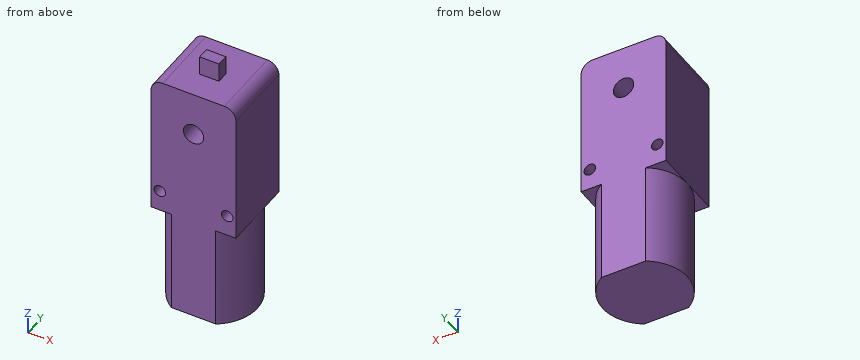
Autodesk Inventor part; units mm, degrees
ref_plane "YZ Plane" through (0, 0, 0) normal (1, 0, 0) x (0, 1, 0)
ref_plane "XZ Plane" through (0, 0, 0) normal (0, 1, 0) x (-1, 0, 0)
ref_plane "XY Plane" through (0, 0, 0) normal (0, 0, 1) x (1, 0, 0)
sketch "Sketch1" plane through (0, 0, 0) normal (0, 1, 0) x (-1, 0, 0)
  line L0 (0, 0) -> (-22, 0)
  line L1 (-22, 0) -> (-22, -37)
  line L2 (-22, -37) -> (0, -37)
  line L3 (0, -37) -> (0, 0)
  line L4 (-11, -37) -> (-11, 0) construction
  circle A0 centre (-11, -11.4) radius 2.65
  circle A1 centre (-19.75, -31.5) radius 1.5
  circle A2 centre (-2.25, -31.5) radius 1.5
  dimension "gearboxWidth" = 22
  dimension "gearboxLength" = 37
  dimension "shaftDiameter" = 5.3
  dimension "shaftCenterToBottom" = 11.4
  dimension "mountHolesDiameter" = 3
  dimension "mountHolesCenterToCenter" = 17.5
  dimension "mountHolesCenterToEdge" = 5.5
extrude "Extrusion1" add sketch "Sketch1" along normal blind 19
sketch "Sketch2" plane through (22, 0, -37) normal (0, 0, -1) x (-1, 0, 0)
  line L0 (0, 19) -> (22, 19)
  line L1 (11, 19) -> (11, 0) construction
  line L2 (0, 0) -> (22, 0)
  ellipse E0 centre (11, 9.5) end of major axis (22, 9.5) minor radius 11.1399 (16.7448, 0) -> (16.7448, 19) ccw
  ellipse E1 centre (11, 9.5) end of major axis (22, 9.5) minor radius 11.1399 (5.2552, 19) -> (5.2552, 0) ccw
  line L3 (5.2552, 19) -> (16.7448, 19)
  line L4 (5.2552, 0) -> (16.7448, 0)
extrude "Extrusion2" add sketch "Sketch2" along normal blind 27
fillet "Fillet1" radius 3 2 edges at (0, 9.5, 0) (22, 9.5, 0)
sketch "Sketch3" plane through (0, 0, 0) normal (0, 0, 1) x (1, 0, 0)
  line L0 (0, 0) -> (22, 0)
  line L1 (16.7448, 0) -> (5.2552, 0)
  line L2 (11, 0) -> (11, 18.9763) construction
  line L3 (8.5, 10) -> (8.5, 7)
  line L4 (8.5, 7) -> (13.5, 7)
  line L5 (13.5, 7) -> (13.5, 10)
  line L6 (13.5, 10) -> (8.5, 10)
  line L7 (8.5, 10) -> (13.5, 7) construction
  line L8 (8.5, 7) -> (13.5, 10) construction
  point P0 (11, 8.5)
  dimension "gearboxTabWidth" = 5
  dimension "gearboxTabHeight" = 3
  dimension "gearboxTabOffsetFromBottom" = 7
extrude "Extrusion3" add sketch "Sketch3" along normal blind 5
properties part number "Yellow_Motor"
Here's how the part is built. I have some questions about the finished solid (model axes, mm). Coordinates: 2 decimals unless noted, no trailing zeros. Order: outer loops, then holes, each group sorted by start corner. A loop starts at its lowest first (then second) coordinate and runs counter-clockwise, first axis right, second up. Notation, with made-up numbers: M 46.5,46.5 L 88.5,46.5 A29 cw 88.5,72.5 Z; hole C -20.75,30 d11. An arc over 180 degrees is marked long. Answer as a JSON object with one key per item and string values. Group by question number.
(1) Suppose I cut it at D-D, the plane x = 6. Please give me the cut outline in (y, z).
(2) For pin 1 (5 mm diameter, centred on x = 16, y = 12, fed in from +Z); pin 2 (2.5 mm diameter, centred on y = 8.5, z = 3, fed in from +X); pin 3 (2.5 mm diameter, centred on x = 2.25, z = -31.5, fed in from +Y); pin 4 (1.5 mm diameter, centred on y = 8.5, z = 2, fed in from -X), each with a flat end and sliding along its axis, tell me the tip position at first contact or that it passes through.
(3) Suppose I cut it at C-C, the plane y = 2.5. State how many separate pieces and enclosed holes the cut face has, then the cut area to 3 significant figures.
(4) Suppose I cut it at A-A, the plane z = -31.5. Please give me the cut outline in (x, y).
(5) Suppose I cut it at B-B, the plane x = 11. Please give me the cut outline in (y, z), then the cut area to 3 significant figures.
(6) I need wall thicknesses on probe 1 along X at (y, z) = (15.75, -11.5); probe 2 along Z at (x, y) = (11, 5.25); probe 3 along Z at (x, y) = (11, 7.25). Which ranges of each line are inside material? Lowest first, please.
Values found:
{
 "1": {"outline": "M 0,-64 L 19,-64 L 19,0 L 0,0 Z"},
 "2": {"pin 1": "stops at z = 0", "pin 2": "stops at x = 13.5", "pin 3": "passes through", "pin 4": "stops at x = 8.5"},
 "3": {"separate pieces": "1", "enclosed holes": "3", "area": "1,240 mm^2"},
 "4": {"outline": "M 0,0 L 0.75,0 L 0.75,19 L 0,19 Z; M 3.75,0 L 18.25,0 L 18.25,19 L 3.75,19 Z; M 21.25,0 L 22,0 L 22,19 L 21.25,19 Z"},
 "5": {"outline": "M 0,-64 L 19,-64 L 19,-14.05 L 0,-14.05 Z; M 0,-8.75 L 19,-8.75 L 19,0 L 10,0 L 10,5 L 7,5 L 7,0 L 0,0 Z", "area": "1,130 mm^2"},
 "6": {"probe 1": "x = 0 to 8.35, 13.65 to 22", "probe 2": "z = -64 to -14.05, -8.75 to 0", "probe 3": "z = -64 to -14.05, -8.75 to 5"}
}
